```python
from build123d import *

# Parameters (mm, degrees)
F0_W     = 21
F0_H     = 6
F2_R     = 4
F3_DEPTH = 100
F4_W     = 5
F4_H     = 5
F5_DEPTH = 5.4
F6_W     = 4.1
F6_H     = 0.2


# Not quite as in the source:
# - a feature names something its author has since deleted; it is built from what else it names


with BuildPart() as f1:
    # F0 (on Front) → F1 (revolve)
    with BuildSketch(Plane.XZ):
        with Locations((10.5, 3)):
            Rectangle(F0_W, F0_H)
    revolve(axis=Axis((0, 0, 3), (0, 0, -1)))

    # F2 (on Top) → F3 (join)
    with BuildSketch(Plane.XY):
        Circle(F2_R)
    extrude(amount=F3_DEPTH)

    # F4 (on face) → F5 (cut)
    with BuildSketch(Plane.XY.offset(6)):
        with Locations((0, 17.8)):
            Rectangle(F4_W, F4_H)
        Polygon((-8.1647553465, 13.1786482665), (-3.5453576839, 15.0920654283), (-5.4587748457, 19.7114630909), (-10.0781725083, 17.7980459291), align=None)
        Polygon((3.5453576839, 15.0920654283), (8.1647553465, 13.1786482665), (10.0781725083, 17.7980459291), (5.4587748457, 19.7114630909), align=None)
        Polygon((9.0509667992, 12.5865007051), (12.5865007051, 9.0509667992), (16.1220346111, 12.5865007051), (12.5865007051, 16.1220346111), align=None)
        Polygon((13.1786482665, 8.1647553465), (15.0920654283, 3.5453576839), (19.7114630909, 5.4587748457), (17.7980459291, 10.0781725083), align=None)
        with Locations((17.8, 0)):
            Rectangle(F4_W, F4_H)
        Polygon((15.0920654283, -3.5453576839), (13.1786482665, -8.1647553465), (17.7980459291, -10.0781725083), (19.7114630909, -5.4587748457), align=None)
        Polygon((12.5865007051, -9.0509667992), (9.0509667992, -12.5865007051), (12.5865007051, -16.1220346111), (16.1220346111, -12.5865007051), align=None)
        Polygon((-12.5865007051, 9.0509667992), (-9.0509667992, 12.5865007051), (-12.5865007051, 16.1220346111), (-16.1220346111, 12.5865007051), align=None)
        Polygon((-15.0920654283, 3.5453576839), (-13.1786482665, 8.1647553465), (-17.7980459291, 10.0781725083), (-19.7114630909, 5.4587748457), align=None)
        with Locations((-17.8, 0)):
            Rectangle(F4_W, F4_H)
        Polygon((-13.1786482665, -8.1647553465), (-15.0920654283, -3.5453576839), (-19.7114630909, -5.4587748457), (-17.7980459291, -10.0781725083), align=None)
        Polygon((-9.0509667992, -12.5865007051), (-12.5865007051, -9.0509667992), (-16.1220346111, -12.5865007051), (-12.5865007051, -16.1220346111), align=None)
        Polygon((-3.5453576839, -15.0920654283), (-8.1647553465, -13.1786482665), (-10.0781725083, -17.7980459291), (-5.4587748457, -19.7114630909), align=None)
        with Locations((0, -17.8)):
            Rectangle(F4_W, F4_H)
        Polygon((8.1647553465, -13.1786482665), (3.5453576839, -15.0920654283), (5.4587748457, -19.7114630909), (10.0781725083, -17.7980459291), align=None)
    extrude(amount=-F5_DEPTH, mode=Mode.SUBTRACT)

    # F6 (on Right) → F7 (revolve)
    with BuildSketch(Plane.YZ):
        with Locations((2.05, 29.9)):
            Rectangle(F6_W, F6_H)
    revolve(axis=Axis((0, 0, 29.9), (0, 0, -1)))


solid = f1.part
```
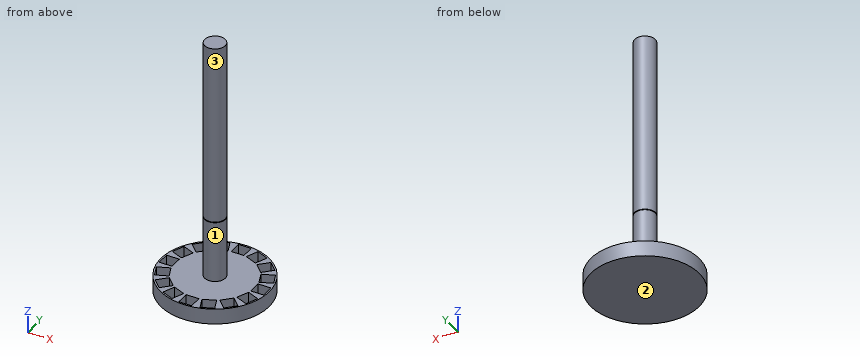
Geometry check sheet. Reference: the model listing, model coordinates, mm. Face numbers are marked on the shaded views. Coordinates: 2 decimals unless noted, no trailing zeros. Write each loop counter-clockwise with the first axis right and the second up, starting at its lowest first coordinate (ties: lowest second). Pieces come first, ordered by that corner, then holes. Notation, with made-up numbers: M 45,15 L 76,15 A22 ccw 76,23 Z; hole C 45,-30.5 d8. An arc over 180 degrees is marked long. Use one line per item in the form item = value. Start each with the question number.
1) Go/stop test with flat-tipped pins: pin 1 Ø1.5 at (x, z) = (-1, 2.5) entering from +Y; pin 2 Ø5.5 at (x, z) = (0.5, 4.5) entering from -Y; pin 3 Ø1.5 at (y, z) = (17, 2) entering from +X; pin 4 Ø1.5 at (x, z) = (6, 81.5) entering from -Y. Record where each tip stops, or that it passes through.
2) Thickness scan on probe 1 along Z at (x, y) = (11, -6.5); probe 2 along Z at (x, y) = (-16.5, 5); probe 3 along Y at (x, z) = (-2.5, 78). Record the ranges inside material, lowest first. Write a range as from..to.
3) Release check for a two-part mould opening along Z. For the marked faces 1, 2 and 3 record: pulls with the +Z half, pulls with the -Z half, needs draft (parallel to the pull), parting line crosses it, or undercut.
4) Section check A-A on x = 0. Enter the section's corners in (y, z).
5) Section check C-C on z = 67.5. Enter the section's corners in (x, y).
Responses:
q1.pin_1 = 21
q1.pin_2 = -21
q1.pin_3 = 13.3
q1.pin_4 = through
q2.probe_1 = 0..6
q2.probe_2 = 0..0.6
q2.probe_3 = -3.12..3.12
q3.face_1 = undercut
q3.face_2 = pulls with the -Z half
q3.face_3 = needs draft
q4.outline = M -21,0 L 21,0 L 21,6 L 20.3,6 L 20.3,0.6 L 15.3,0.6 L 15.3,6 L 4,6 L 4,29.8 L 4.1,29.8 L 4.1,30 L 4,30 L 4,100 L -4,100 L -4,30 L -4.1,30 L -4.1,29.8 L -4,29.8 L -4,6 L -15.3,6 L -15.3,0.6 L -20.3,0.6 L -20.3,6 L -21,6 Z
q5.outline = C 0,0 d8
